```python
from build123d import *

# Parameters (mm, degrees)
F0_W      = 63.5
F0_H      = 31.75
F1_DEPTH  = 6.35
F2_W      = 4.7625
F2_H      = 6.35
F3_DEPTH  = 12.7
F4_W      = 4.7625
F4_H      = 6.35
F5_DEPTH  = 12.7
F6_W      = 4.7625
F6_H      = 12.7
F7_DEPTH  = 5.08
F8_R      = 3.571875
F8_R_2    = 0.9615286486
F9_DEPTH  = 2.38125
F10_DEPTH = 6.35
F11_W     = 4.7625
F11_H     = 12.7
F12_DEPTH = 5.08
F13_R     = 0.9615297
F14_DEPTH = 6.35
F13_R_2   = 3.571875
F15_DEPTH = 2.38125
F16_DEPTH = 31.75
F17_DEPTH = 3.175
F18_W     = 3.175
F18_H     = 31.75
F19_DEPTH = 6.35


with BuildPart() as f1:
    # F0 (on Front) → F1 (new body)
    with BuildSketch(Plane.XZ):
        with Locations((-31.75, 54.4051597416)):
            Rectangle(F0_W, F0_H)
    extrude(amount=F1_DEPTH)

    # F2 (on face) → F3 (join)
    with BuildSketch(Plane.XY.offset(70.2801597416)):
        with Locations((-61.11875, -3.175)):
            Rectangle(F2_W, F2_H)
    extrude(amount=F3_DEPTH)

    # F4 (on face) → F5 (join)
    with BuildSketch(Plane(origin=(0, 0, 38.5301597416), x_dir=(1, 0, 0), z_dir=(0, 0, -1))):
        with Locations((-61.11875, 3.175)):
            Rectangle(F4_W, F4_H)
    extrude(amount=F5_DEPTH)

    # F6 (on face) → F7 (join)
    with BuildSketch(Plane(origin=(0, 0, 0), x_dir=(-1, 0, 0), z_dir=(0, 1, 0))):
        with Locations((61.11875, 76.6301597416)):
            Rectangle(F6_W, F6_H)
    extrude(amount=F7_DEPTH)

    # F8 (on face) → F9 (cut)
    with BuildSketch(Plane.YZ.offset(-58.7375)):
        with Locations((-0.5586565495, 77.6017636912)):
            Circle(F8_R)
        with Locations((-0.5586565495, 77.6017636912)):
            Circle(F8_R_2, mode=Mode.SUBTRACT)
    extrude(amount=-F9_DEPTH, mode=Mode.SUBTRACT)

    # F8 (on face) → F10 (cut)
    with BuildSketch(Plane.YZ.offset(-58.7375)):
        with Locations((-0.5586565495, 77.6017636912)):
            Circle(F8_R_2)
    extrude(amount=-F10_DEPTH, mode=Mode.SUBTRACT)

    # F11 (on face) → F12 (join)
    with BuildSketch(Plane(origin=(0, 0, 0), x_dir=(-1, 0, 0), z_dir=(0, 1, 0))):
        with Locations((61.11875, 32.1801597416)):
            Rectangle(F11_W, F11_H)
    extrude(amount=F12_DEPTH)

    # F13 (on face) → F14 (cut)
    with BuildSketch(Plane.YZ.offset(-58.7375)):
        with Locations((-0.6811455784, 31.2418671489)):
            Circle(F13_R)
    extrude(amount=-F14_DEPTH, mode=Mode.SUBTRACT)

    # F13 (on face) → F15 (cut)
    with BuildSketch(Plane.YZ.offset(-58.7375)):
        with Locations((-0.6811455784, 31.2418671489)):
            Circle(F13_R_2)
        with Locations((-0.6811455784, 31.2418671489)):
            Circle(F13_R, mode=Mode.SUBTRACT)
    extrude(amount=-F15_DEPTH, mode=Mode.SUBTRACT)

    # F16 (add): a face of the model
    f16_faces = [f1.faces().sort_by_distance(p)[0] for p in [
        (-61.11875, 2.54, 70.2801597416),
    ]]
    extrude(f16_faces, amount=F16_DEPTH)

    # F17 (add): a face of the model
    f17_faces = [f1.faces().sort_by_distance(p)[0] for p in [
        (0, -3.175, 54.4051597416),
    ]]
    extrude(f17_faces, amount=F17_DEPTH)

    # F18 (on face) → F19 (join)
    with BuildSketch(Plane.XZ.offset(6.35)):
        with Locations((1.5875, 54.4051597416)):
            Rectangle(F18_W, F18_H)
    extrude(amount=F19_DEPTH)


solid = f1.part
```
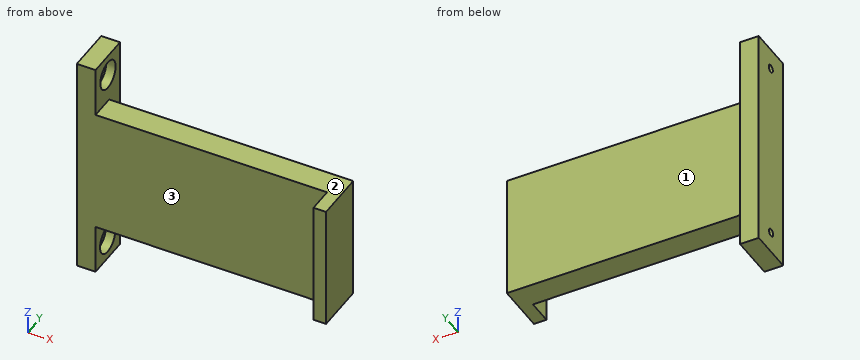
CAD build for the part. Positions are in the model's coordinates, mm. Face numbers are marked on the shaded views. A direction names the side the tool comes from. Coordinates: 2 decimals unless noted, no trailing zeros. Order: outer loops, then holes, each group sorted by start corner. A loop starts at its lowest first (then second) coordinate and runs counter-clockwise, first axis right, second up. Notation, with made-up numbers: (65, 88) - (72, 88) arc R12 ccw to (72, 100) - close; hole circle Ø11 at (-19.75, 32). An arc over 180 degrees is marked (long way). Use a Markdown table: item, result. Add a question column.
(1) Saw through at B-B (y = -3). Give the cut face in (x, z) (1 decimal), then the cut area to 3 significant figures.
(2) Saw through at C-C (x = -46). Give the cut face in (y, z).
(3) Drill centre lines: line 1 along X through (y, z) = (-10.5, 45.5) (3 decimals); line 2 along Y through (x, z) = (-38.5, 62.5); line 3 along X through (y, z) = (3.75, 77). Where is each one in solid material? Low to high. Write a range as [from, to].
(4) Which spindle directions (+Z, -Z, +X, -X, +Y, -Y) get a long thin tool onto all of the face, cutting with end or side? Do the marked faces 1, 2 and 3. Say none if no direction does.
(5) Flat gauge pins, fed straight in: pin 1 (10 mm diameter, centred on x = -33.5, y = -8, fed in from +Z); pin 2 (10 mm diameter, centred on x = -10, z = 74.5, fed in from +Y); pin 3 (8 mm diameter, centred on y = -0.56, z = 77.6, fed in from +X). Where does each tip first touch, or does it go through?
(6) Saw through at D-D (y = 2). Give the cut face in (x, z).
Solved:
| question | item | result |
|---|---|---|
| 1 | outline | (-63.5, 25.8) - (-58.7, 25.8) - (-58.7, 28.5) - (-61.1, 28.5) - (-61.1, 34) - (-58.7, 34) - (-58.7, 38.5) - (3.2, 38.5) - (3.2, 70.3) - (-58.7, 70.3) - (-58.7, 75) - (-61.1, 75) - (-61.1, 80.2) - (-58.7, 80.2) - (-58.7, 83) - (-63.5, 83) - close |
| 1 | area | 2,210 mm² |
| 2 | outline | (-6.35, 38.53) - (0, 38.53) - (0, 70.28) - (-6.35, 70.28) - close |
| 3 | line 1 | x = [0, 3.175] |
| 3 | line 2 | y = [-6.35, 0] |
| 3 | line 3 | x = [-63.5, -58.74] |
| 4 | face 1 | +Z, -Z, +X, +Y |
| 4 | face 2 | +Z, +X, +Y, -Y |
| 4 | face 3 | +Z, -Z, -X, -Y |
| 5 | pin 1 | stops at z = 70.28 |
| 5 | pin 2 | stops at y = 0 |
| 5 | pin 3 | stops at x = -58.74 |
| 6 | outline | (-63.5, 25.83) - (-58.74, 25.83) - (-58.74, 28.88) - (-61.12, 28.88) - (-61.12, 33.6) - (-58.74, 33.6) - (-58.74, 75.11) - (-61.12, 75.11) - (-61.12, 80.09) - (-58.74, 80.09) - (-58.74, 82.98) - (-63.5, 82.98) - close |
